CAD build for the part. Positions are in the model's coordinates, mm. A direction names the side the tool comes from. Give positions to 0.01 mm unless a question says otherwise; leave off trailing zeros. Write each loop counter-clockwise with the first axis right and the second up, starting at its lowest first coordinate (ties: lowest second). Pieces come first, ordered by that corner, then holes. Notation, with made-up numbers: (75.5, 29.25) -> (81.5, 29.25) arc R12 cw to (81.5, 48.25) -> close; hole circle Ø2 at (86, 86). An arc over 180 degrees is marked (long way). Use one line per item in the form item = value. Start each with the question number.
from build123d import *

# Parameters (mm, degrees)
F1_DEPTH = 0.3
F3_DEPTH = 3.2
F4_R     = 0.2
F5_R     = 0.225
F6_DEPTH = 3


with BuildPart() as f1:
    # F0 (on Top) → F1 (new body)
    with BuildSketch(Plane.XY):
        with BuildLine():
            Line((3.2, 2.35), (-3.2, 2.35))
            ThreePointArc((-3.2, 2.35), (-5.55, 0), (-3.2, -2.35))
            Line((-3.2, -2.35), (3.2, -2.35))
            ThreePointArc((3.2, -2.35), (5.55, 0), (3.2, 2.35))
        make_face()
    extrude(amount=F1_DEPTH)

    # F2 (on face) → F3 (join)
    with BuildSketch(Plane.XY.offset(0.3)):
        with BuildLine():
            Line((3.2, 1.95), (-3.2, 1.95))
            ThreePointArc((-3.2, 1.95), (-5.15, 0), (-3.2, -1.95))
            Line((-3.2, -1.95), (3.2, -1.95))
            ThreePointArc((3.2, -1.95), (5.15, 0), (3.2, 1.95))
        make_face()
    extrude(amount=F3_DEPTH)

    # F4
    f4_edges = [f1.edges().sort_by_distance(p)[0] for p in [
        (0, 1.95, 3.5),
        (-5.15, 0, 3.5),
        (0, -1.95, 3.5),
        (5.15, 0, 3.5),
    ]]
    fillet(f4_edges, radius=F4_R)

    # F5 (on face) → F6 (join)
    with BuildSketch(Plane(origin=(0, 0, 0), x_dir=(1, 0, 0), z_dir=(0, 0, -1))):
        with Locations((-2.44, 0)):
            Circle(F5_R)
        with Locations((2.44, 0)):
            Circle(F5_R)
    extrude(amount=F6_DEPTH)


solid = f1.part
1) Wall check: line 1 along Z through (x, y) = (1.25, -1.1); line 2 along Y through (x, z) = (1, 2.25); line 3 along X through (y, z) = (0.1, -0.25). Give the ranges that are in metal, low to high. Write a range as from..to.
2) Cut at A-A (x = -2.44). Give the cut face in (y, z) (3 decimals).
3) Cut at D-D (x = 1.25). Give the cut face in (y, z), and give its area (3 significant figures).
4) Pin check, flat tips, straight feed: pin 1 (1.5 mm diameter, centred on x = 1.5, z = 1.5, fed in from -Y); pin 2 (1.5 mm diameter, centred on x = -3.5, y = -1, fed in from -Z); pin 3 (1.5 mm diameter, centred on y = 0.5, z = 1, fed in from +X). Stop position of each tip, or through.
5) Cut at B-B (y = 0). Give the cut face in (x, z) (3 decimals).
6) 3-axis set-ups, long thin cutter, end or side, ignore diameter. For faces 1 (the face through (0, -1.95, 2)), 2 (the face through (0, -2.1, 0.3)), 3 (the face through (-5.15, 0.04, 1.78)), 4 (the face through (5.15, -0.04, 1.78)): which of +Z, -Z, +X, -X, +Y, -Y reach the whole face in a straight line?
7) Cut at C-C (z = 1.5). Give the cut face in (x, y).
Final values:
q1.line_1 = 0..3.5
q1.line_2 = -1.95..1.95
q1.line_3 = -2.64..-2.24, 2.24..2.64
q2.outline = (-2.35, 0) -> (-0.225, 0) -> (-0.225, -3) -> (0.225, -3) -> (0.225, 0) -> (2.35, 0) -> (2.35, 0.3) -> (1.95, 0.3) -> (1.95, 3.3) arc R0.2 ccw to (1.75, 3.5) -> (-1.75, 3.5) arc R0.2 ccw to (-1.95, 3.3) -> (-1.95, 0.3) -> (-2.35, 0.3) -> close
q3.outline = (-2.35, 0) -> (2.35, 0) -> (2.35, 0.3) -> (1.95, 0.3) -> (1.95, 3.3) arc R0.2 ccw to (1.75, 3.5) -> (-1.75, 3.5) arc R0.2 ccw to (-1.95, 3.3) -> (-1.95, 0.3) -> (-2.35, 0.3) -> close
q3.area = 13.9 mm^2
q4.pin_1 = -1.95
q4.pin_2 = 0
q4.pin_3 = 5.54
q5.outline = (-5.55, 0) -> (-2.665, 0) -> (-2.665, -3) -> (-2.215, -3) -> (-2.215, 0) -> (2.215, 0) -> (2.215, -3) -> (2.665, -3) -> (2.665, 0) -> (5.55, 0) -> (5.55, 0.3) -> (5.15, 0.3) -> (5.15, 3.3) arc R0.2 ccw to (4.95, 3.5) -> (-4.95, 3.5) arc R0.2 ccw to (-5.15, 3.3) -> (-5.15, 0.3) -> (-5.55, 0.3) -> close
q6.face_1 = +Z, +X, -X, -Y
q6.face_2 = +Z
q6.face_3 = +Z, -X
q6.face_4 = +Z, +X
q7.outline = (-3.2, -1.95) -> (3.2, -1.95) arc R1.95 ccw to (3.2, 1.95) -> (-3.2, 1.95) arc R1.95 ccw to start
